Can you work these out from the model? Positions are in its coordinate system, mm. A direction names the side the tool comes from. Coordinates: 2 decimals unless noted, no trailing zeros. Order: outer loops, then holes, each group sorted by start corner. A loop starts at its lowest first (then second) coordinate and runs counter-clockwise, first axis right, second up.
Autodesk Fusion 360 part; units mm, degrees
sketch "Sketch1" plane through (0, 0, 0) normal (0, 1, 0) x (1, 0, 0)
  line L0 (0, 0) -> (115, 0)
  line L1 (115, -70) -> (0, -70)
  ellipse E0 centre (0, -35) end of major axis (0, -70) minor radius 20 (0, 0) -> (0, -70) ccw
  ellipse E1 centre (115, -35) end of major axis (115, -70) minor radius 20 (115, -70) -> (115, 0) ccw
  circle A0 centre (-10, -35) radius 2.5
  circle A1 centre (125, -35) radius 2.5
  dimension "d1" = 20
  dimension "d2" = 5
  dimension "d3" = 10
extrude "Extrude1" add sketch "Sketch1" along normal blind 1
sketch "Sketch3" plane through (0, 0, 0) normal (0, -1, 0) x (1, 0, 0)
  circle A0 centre (-10, 35) radius 2.5
  circle A1 centre (125, 35) radius 2.5
  ellipse E0 centre (0, 35) end of major axis (0, 70) minor radius 20 (0, 70) -> (0, 0) ccw
  line L0 (0, 0) -> (115, 0)
  ellipse E1 centre (115, 35) end of major axis (115, 70) minor radius 20 (115, 0) -> (115, 70) ccw
  line L1 (115, 70) -> (0, 70)
  line L2 (0, 1) -> (115, 1)
  spline S0 degree 3 poles (115, 1) (118.1745, 1) (121.3862, 2.4713) (124.2603, 5.3633) (127.2867, 8.4088) (129.8847, 13.0253) (131.6024, 18.5351) (133.5298, 24.7176) (134.3377, 31.9986) (133.8651, 39.0248) (133.4191, 45.6553) (131.8372, 52.0318) (129.4075, 57.0895) (127.2109, 61.662) (124.3332, 65.1363) (121.2436, 67.0835) (119.2133, 68.3631) (117.1029, 69) (115, 69) knots 3.141593 3.141593 3.141593 3.141593 3.663435 3.663435 3.663435 4.212955 4.212955 4.212955 4.82957 4.82957 4.82957 5.411454 5.411454 5.411454 5.937501 5.937501 5.937501 6.283185 6.283185 6.283185 6.283185
  line L3 (115, 69) -> (0, 69)
  spline S1 degree 3 poles (0, 69) (-3.1745, 69) (-6.3862, 67.5287) (-9.2603, 64.6367) (-12.2867, 61.5912) (-14.8847, 56.9747) (-16.6024, 51.4649) (-18.5298, 45.2824) (-19.3377, 38.0014) (-18.8651, 30.9752) (-18.4191, 24.3447) (-16.8372, 17.9682) (-14.4075, 12.9105) (-12.2109, 8.338) (-9.3332, 4.8637) (-6.2436, 2.9165) (-4.2133, 1.6369) (-2.1029, 1) (0, 1) knots 0 0 0 0 0.521842 0.521842 0.521842 1.071362 1.071362 1.071362 1.687978 1.687978 1.687978 2.269861 2.269861 2.269861 2.795908 2.795908 2.795908 3.141593 3.141593 3.141593 3.141593
  dimension "d6" = -1
extrude "Extrude2" add sketch "Sketch3" along normal blind 4 contours E0 L0 E1 L1
sketch "Sketch4" plane through (0, 0, 0) normal (0, 1, 0) x (1, 0, 0)
  line L0 (3.55, -65.5) -> (110.65, -65.5)
  line L1 (110.65, -65.5) -> (110.65, -4.5)
  line L2 (110.65, -4.5) -> (3.55, -4.5)
  line L3 (3.55, -4.5) -> (3.55, -65.5)
  line L4 (115, -1) -> (0, -1)
  line L5 (1, -67) -> (113, -67)
  line L6 (113, -67) -> (113, -3)
  line L7 (113, -3) -> (1, -3)
  line L8 (1, -3) -> (1, -67)
  point P0 (0, -35)
  dimension "d9" = 61
  dimension "d10" = 107.1
  dimension "d11" = 3.55
  dimension "d12" = 3.5
extrude "Extrude3" add sketch "Sketch4" against normal blind 2
sketch "Sketch5" plane through (0, 0, 0) normal (0, 1, 0) x (-1, 0, 0)
  line L0 (-4.5848, 64.4333) -> (-109.4505, 64.4333)
  line L1 (-109.4505, 64.4333) -> (-109.4505, 5.2457)
  line L2 (-109.4505, 5.2457) -> (-4.5848, 5.2457)
  line L3 (-4.5848, 5.2457) -> (-4.5848, 64.4333)
extrude "Extrude4" cut sketch "Sketch5" along normal blind 10
sketch "Sketch6" plane through (1, 0, 0) normal (-1, 0, 0) x (0, -1, 0)
  line L0 (0, 67) -> (0, 3)
  line L1 (0, 3) -> (2, 3)
  line L2 (2, 3) -> (2, 67)
  line L3 (2, 67) -> (0, 67)
  line L4 (-3, 27) -> (6, 27)
  line L5 (6, 27) -> (6, 20)
  line L6 (6, 20) -> (-3, 20)
  line L7 (-3, 20) -> (-3, 27)
  line L8 (0, 35) -> (9, 35)
  line L9 (-3, 43) -> (6, 43)
  line L10 (6, 43) -> (6, 50)
  line L11 (6, 50) -> (-3, 50)
  line L12 (-3, 50) -> (-3, 43)
extrude "Extrude5" cut sketch "Sketch6" along normal blind 30 contours L0 L2 L9 L11 | L2 L9 L10 L11
extrude "Extrude6" cut sketch "Sketch6" against normal blind 9 contours L0 L2 L9 L11 | L2 L9 L10 L11
extrude "Extrude7" cut sketch "Sketch6" along normal blind 30 contours L0 L2 L4 L6 | L2 L4 L5 L6
extrude "Extrude8" cut sketch "Sketch6" against normal blind 10 contours L0 L2 L4 L6 | L2 L4 L5 L6
1. I'm going to push flat-ended pins straight in: pin 1 (1 mm diameter, centred on y = -0.5, z = 25, fed in from +X); pin 2 (3 mm diameter, centred on x = 2, z = 45, fed in from -Y); pin 3 (2 mm diameter, centred on x = 2.5, z = 33.5, fed in from -Y). Where does each tip first touch, or does it pass through?
Completed:
pin 1: stops at x = 134.25
pin 2: stops at y = 0
pin 3: stops at y = -2
2. Please list where these lines run through material, in increasing order: probe 1 along X at (y, z) = (0.35, 35); probe 2 along Z at (x, y) = (46.5, -0.6); probe 3 along Z at (x, y) = (103, 0.1).
Completed:
probe 1: x = -20 to -12.5, -7.5 to 4.58, 109.45 to 122.5, 127.5 to 135
probe 2: z = 0 to 1, 3 to 4.5, 65.5 to 67, 69 to 70
probe 3: z = 0 to 5.25, 64.43 to 70
3. On a 3-axis mill with a long thin cutter (end or side, diameter ignored), from which of +Z, -Z, +X, -X, +Y, -Y can I reach the whole of each face in a straight line? I mean faces 1 (the flat face through (57, -2, 1)), 2 (the cylindrical face through (127.385, 0.493, 35.751)). Say none if no direction works.
Completed:
face 1: -Y
face 2: +Y, -Y
4. Imagine slicing it at B-B on z = 35. Give the number of separate pieces and of enclosed holes in the cut face, then the cut area to 3 significant figures.
Completed:
separate pieces: 4
enclosed holes: 0
area: 58.0 mm2
5. Imagine slicing it at A-A on x = 75. Please give me the cut outline in (y, z).
Completed:
outline: (-4, 0) - (1, 0) - (1, 5.25) - (0, 5.25) - (0, 4.5) - (-2, 4.5) - (-2, 3) - (0, 3) - (0, 1) - (-4, 1) - close; (-4, 69) - (0, 69) - (0, 67) - (-2, 67) - (-2, 65.5) - (0, 65.5) - (0, 64.43) - (1, 64.43) - (1, 70) - (-4, 70) - close
6. Thinking about a two-plate mould opening in Z: for faces 3 (the flat face through (58, -2, 69)), 4 (the flat face through (57, -2, 0)), 5 (the flat face through (65, -2, 66)), 6 (the flat face through (57, 1, 4)), which applies, pulls with the +Z half, pulls with the -Z half, needs draft (parallel to the pull), parting line crosses it, or undercut?
Completed:
face 3: undercut
face 4: pulls with the -Z half
face 5: undercut
face 6: needs draft
